from build123d import *

# Parameters (mm, degrees)
SKIZZE1_R                       = 22.5
AUFSATZ_LINEAR_AUSTRAGEN1_DEPTH = 15
SKIZZE2_R                       = 16
AUFSATZ_LINEAR_AUSTRAGEN2_DEPTH = 2
SKIZZE3_R                       = 10
SCHNITT_LINEAR_AUSTRAGEN1_DEPTH = 37.076308015
SKIZZE7_R                       = 2.75
SCHNITT_LINEAR_AUSTRAGEN2_DEPTH = 37.076308015


with BuildPart() as part:
    # Skizze1 → Aufsatz-Linear austragen1 (new body)
    with BuildSketch(Plane.XY):
        Circle(SKIZZE1_R)
    extrude(amount=AUFSATZ_LINEAR_AUSTRAGEN1_DEPTH)

    # Skizze2 → Aufsatz-Linear austragen2 (add)
    with BuildSketch(Plane(origin=(0, 0, 0), x_dir=(-1, 0, 0), z_dir=(0, 0, -1))):
        Circle(SKIZZE2_R)
    extrude(amount=AUFSATZ_LINEAR_AUSTRAGEN2_DEPTH)

    # Skizze3 → Schnitt-Linear austragen1 (cut, through all)
    with BuildSketch(Plane(origin=(0, 0, -2), x_dir=(-1, 0, 0), z_dir=(0, 0, -1))):
        Circle(SKIZZE3_R)
    extrude(amount=-SCHNITT_LINEAR_AUSTRAGEN1_DEPTH, mode=Mode.SUBTRACT)

    # Skizze7 → Schnitt-Linear austragen2 (cut, through all)
    with BuildSketch(Plane(origin=(0, 0, -2), x_dir=(-1, 0, 0), z_dir=(0, 0, -1))):
        with Locations((0, 15.25)):
            Circle(SKIZZE7_R)
        with Locations((15.25, 0)):
            Circle(SKIZZE7_R)
        with Locations((0, -15.25)):
            Circle(SKIZZE7_R)
        with Locations((-15.25, 0)):
            Circle(SKIZZE7_R)
    extrude(amount=-SCHNITT_LINEAR_AUSTRAGEN2_DEPTH, mode=Mode.SUBTRACT)


solid = part.part
Could you check a few things on this model? Use its own coordinates, in mm. A direction names the side the tool comes from. Give positions to 0.01 mm unless a question says otherwise; leave off trailing zeros. Loops run counter-clockwise (first coordinate to the right, second up) from the corner with the lowest first, then second, coordinate; pieces in that order, holes last. Notation, with made-up numbers: M 21,-26.75 L 79,-26.75 A16 cw 79,3.25 Z; hole C 24.25,72.25 d8. An arc over 180 degrees is marked long. Answer as a JSON object with one key per item and string values.
Q1. Suppose I cut it at B-B, the plane y = 6. List the corners of the cut face in (x, z) for me.
Values found:
{"outline": "M -21.69,0 L -14.83,0 L -14.83,-2 L -8,-2 L -8,15 L -21.69,15 Z; M 8,-2 L 14.83,-2 L 14.83,0 L 21.69,0 L 21.69,15 L 8,15 Z"}
Q2. Suppose I cut it at A-A, the plane x = 0. List the corners of the cut face in (y, z) for me.
Values found:
{"outline": "M -22.5,0 L -18,0 L -18,15 L -22.5,15 Z; M -12.5,-2 L -10,-2 L -10,15 L -12.5,15 Z; M 10,-2 L 12.5,-2 L 12.5,15 L 10,15 Z; M 18,0 L 22.5,0 L 22.5,15 L 18,15 Z"}
Q3. If I drill on probe 1 along Y at (x, z) = (0, 9.5); probe 2 along X at (y, z) = (-0.5, 1.75); probe 3 along Y at (x, z) = (15.25, 3.75), over which ranges is the centre line in solid material (lowest first)? Write a range as [from, to].
Values found:
{"probe 1": "y = [-22.5, -18], [-12.5, -10], [10, 12.5], [18, 22.5]", "probe 2": "x = [-22.49, -17.95], [-12.55, -9.99], [9.99, 12.55], [17.95, 22.49]", "probe 3": "y = [-16.54, -2.75], [2.75, 16.54]"}
Q4. For faces 4 (the cylindrical face through (0.596, 12.565, 6.381)), 5 (the cylindrical face through (11.411, -11.216, -0.986)), 6 (the cylindrical face through (11.216, 11.411, -0.986)), 7 (the cylindrical face through (-11.411, 11.216, -0.986)), 8 (the flat face through (-5.3, 15.3, 0)), which set-ups out of +Z, -Z, +X, -X, +Y, -Y let a thin tool reach every point of the face, with its end or its side?
Values found:
{"face 4": "+Z, -Z", "face 5": "-Z, +X, -Y", "face 6": "-Z, +X, +Y", "face 7": "-Z, -X, +Y", "face 8": "-Z"}
Q5. Suppose I cut it at C-C, the plane z = 4.25. List the corners of the cut face in (x, y) for me, plus the area to 3 significant figures.
Values found:
{"outline": "C 0,0 d45; hole C -15.25,0 d5.5; hole C 0,0 d20; hole C 0,-15.25 d5.5; hole C 0,15.25 d5.5; hole C 15.25,0 d5.5", "area": "1,180 mm²"}
Q6. For P1, Ø1.5, axis at y = 9.5, z = 10.5, coming from the +X side; P2, Ø12, axis at x = 0, y = 0, coming from the +Z side; P3, Ø3, axis at x = -17.5, z = 11.5, coming from the +Y side; P4, Ø22.5, axis at x = 4.5, y = 2, coming from the -Z side, each with a flat end and sliding along its axis, tell me the tip position at first contact or that it passes through.
Values found:
{"P1": "stops at x = 20.73", "P2": "passes through", "P3": "stops at y = 15.82", "P4": "stops at z = -2"}
Q7. If we mould it in two halves opening along X, with no side actions, what happens to faces 1 (the cylindrical face through (10.382, -19.961, 7.395)), 2 (the cylindrical face through (-12.5, 0.1, 6.4)), 3 (the cylindrical face through (-11.216, -11.411, -0.986))? For each: pulls with the +X half, pulls with the -X half, needs draft (parallel to the pull), parting line crosses it, or undercut.
Values found:
{"face 1": "parting line crosses it", "face 2": "undercut", "face 3": "pulls with the -X half"}
